```python
from build123d import *

# Parameters (mm, degrees)
BOSS_EXTRUDE1_DEPTH = 4


with BuildPart() as part:
    # Sketch2 → Boss-Extrude1 (new body)
    with BuildSketch(Plane.XY):
        with BuildLine():
            Line((-138.118918248, -4), (-138.118918248, -8))
            Line((-138.118918248, -8), (-118.118918248, -8))
            Line((-118.118918248, -8), (-118.118918248, -4))
            Line((-118.118918248, -4), (-78.118918248, -4))
            Line((-78.118918248, -4), (-78.118918248, -8))
            Line((-78.118918248, -8), (-18.118918248, -8))
            Line((-18.118918248, -8), (-18.118918248, -4))
            Line((-18.118918248, -4), (21.881081752, -4))
            Line((21.881081752, -4), (21.881081752, -8))
            Line((21.881081752, -8), (81.881081752, -8))
            Line((81.881081752, -8), (81.881081752, -4))
            Line((81.881081752, -4), (121.881081752, -4))
            Line((121.881081752, -4), (121.881081752, -8))
            Line((121.881081752, -8), (141.881081752, -8))
            Line((141.881081752, -8), (141.881081752, -4))
            Line((141.881081752, -4), (126.420932439, 77))
            Line((126.420932439, 77), (121.881081752, 77))
            Line((121.881081752, 77), (121.881081752, 47))
            Line((121.881081752, 47), (117.881081752, 47))
            Line((117.881081752, 47), (117.881081752, 77))
            Line((117.881081752, 77), (113.803791589, 77))
            Line((113.803791589, 77), (105.805256721, 36.507417232))
            ThreePointArc((105.805256721, 36.507417232), (101.881081752, 33.282562905), (97.956906783, 36.507417232))
            Line((97.956906783, 36.507417232), (89.958371916, 77))
            Line((89.958371916, 77), (85.881081752, 77))
            Line((85.881081752, 77), (85.881081752, 47))
            Line((85.881081752, 47), (81.881081752, 47))
            Line((81.881081752, 47), (81.881081752, 77))
            Line((81.881081752, 77), (21.881081752, 77))
            Line((21.881081752, 77), (21.881081752, 47))
            Line((21.881081752, 47), (17.881081752, 47))
            Line((17.881081752, 47), (17.881081752, 77))
            Line((17.881081752, 77), (-14.118918248, 77))
            Line((-14.118918248, 77), (-14.118918248, 47))
            Line((-14.118918248, 47), (-18.118918248, 47))
            Line((-18.118918248, 47), (-18.118918248, 77))
            Line((-18.118918248, 77), (-78.118918248, 77))
            Line((-78.118918248, 77), (-78.118918248, 47))
            Line((-78.118918248, 47), (-82.118918248, 47))
            Line((-82.118918248, 47), (-82.118918248, 77))
            Line((-82.118918248, 77), (-86.196208411, 77))
            Line((-86.196208411, 77), (-94.194743279, 36.507417232))
            ThreePointArc((-94.194743279, 36.507417232), (-98.118918248, 33.282562905), (-102.043093217, 36.507417232))
            Line((-102.043093217, 36.507417232), (-110.041628084, 77))
            Line((-110.041628084, 77), (-114.118918248, 77))
            Line((-114.118918248, 77), (-114.118918248, 47))
            Line((-114.118918248, 47), (-118.118918248, 47))
            Line((-118.118918248, 47), (-118.118918248, 77))
            Line((-118.118918248, 77), (-122.658768935, 77))
            Line((-122.658768935, 77), (-138.118918248, -4))
        make_face()
        with BuildLine():
            Line((-102.438497969, 0), (-93.799338527, 0))
            ThreePointArc((-93.799338527, 0), (-90.499180816, 1.739699338), (-90.069664197, 5.445520459))
            Line((-90.069664197, 5.445520459), (-94.389243919, 16.590728056))
            ThreePointArc((-94.389243919, 16.590728056), (-98.118918248, 19.145207598), (-101.848592577, 16.590728056))
            Line((-101.848592577, 16.590728056), (-106.168172299, 5.445520459))
            ThreePointArc((-106.168172299, 5.445520459), (-105.73865568, 1.739699338), (-102.438497969, 0))
        make_face(mode=Mode.SUBTRACT)
        with BuildLine():
            Line((-22.118918248, 4), (-22.118918248, 52.759761907))
            ThreePointArc((-22.118918248, 52.759761907), (-24.865306485, 56.558242859), (-29.333147021, 55.140672109))
            Line((-29.333147021, 55.140672109), (-65.451489175, 6.380910203))
            ThreePointArc((-65.451489175, 6.380910203), (-65.80962942, 2.200505739), (-62.237260401, 0))
            Line((-62.237260401, 0), (-26.118918248, 0))
            ThreePointArc((-26.118918248, 0), (-23.290491123, 1.171572875), (-22.118918248, 4))
        make_face(mode=Mode.SUBTRACT)
        with BuildLine():
            Line((-34.000576095, 73), (-70.118918248, 73))
            ThreePointArc((-70.118918248, 73), (-72.947345373, 71.828427125), (-74.118918248, 69))
            Line((-74.118918248, 69), (-74.118918248, 20.240238093))
            ThreePointArc((-74.118918248, 20.240238093), (-71.372530011, 16.441757141), (-66.904689475, 17.859327891))
            Line((-66.904689475, 17.859327891), (-30.786347321, 66.619089797))
            ThreePointArc((-30.786347321, 66.619089797), (-30.428207076, 70.799494261), (-34.000576095, 73))
        make_face(mode=Mode.SUBTRACT)
        with BuildLine():
            Line((9.881081752, 73), (-2.356754744, 73))
            ThreePointArc((-2.356754744, 73), (-5.664234687, 71.249572499), (-6.076962704, 67.530288213))
            Line((-6.076962704, 67.530288213), (6.160873792, 36.553264583))
            ThreePointArc((6.160873792, 36.553264583), (10.62913528, 34.093546905), (13.881081752, 38.02297637))
            Line((13.881081752, 38.02297637), (13.881081752, 69))
            ThreePointArc((13.881081752, 69), (12.709508877, 71.828427125), (9.881081752, 73))
        make_face(mode=Mode.SUBTRACT)
        with BuildLine():
            Line((-6.118918248, 0), (6.118918248, 0))
            ThreePointArc((6.118918248, 0), (9.426398191, 1.750427501), (9.839126208, 5.469711787))
            Line((9.839126208, 5.469711787), (-2.398710288, 36.446735417))
            ThreePointArc((-2.398710288, 36.446735417), (-6.866971776, 38.906453095), (-10.118918248, 34.97702363))
            Line((-10.118918248, 34.97702363), (-10.118918248, 4))
            ThreePointArc((-10.118918248, 4), (-8.947345373, 1.171572875), (-6.118918248, 0))
        make_face(mode=Mode.SUBTRACT)
        with BuildLine():
            Line((105.610756081, 16.590728056), (109.930335803, 5.445520459))
            ThreePointArc((109.930335803, 5.445520459), (109.500819184, 1.739699338), (106.200661473, 0))
            Line((106.200661473, 0), (97.561502031, 0))
            ThreePointArc((97.561502031, 0), (94.26134432, 1.739699338), (93.831827701, 5.445520459))
            Line((93.831827701, 5.445520459), (98.151407423, 16.590728056))
            ThreePointArc((98.151407423, 16.590728056), (101.881081752, 19.145207598), (105.610756081, 16.590728056))
        make_face(mode=Mode.SUBTRACT)
        with BuildLine():
            Line((70.666852979, 17.859327891), (34.548510825, 66.619089797))
            ThreePointArc((34.548510825, 66.619089797), (34.19037058, 70.799494261), (37.762739599, 73))
            Line((37.762739599, 73), (73.881081752, 73))
            ThreePointArc((73.881081752, 73), (76.709508877, 71.828427125), (77.881081752, 69))
            Line((77.881081752, 69), (77.881081752, 20.240238093))
            ThreePointArc((77.881081752, 20.240238093), (75.134693515, 16.441757141), (70.666852979, 17.859327891))
        make_face(mode=Mode.SUBTRACT)
        with BuildLine():
            Line((65.999423905, 0), (29.881081752, 0))
            ThreePointArc((29.881081752, 0), (27.052654627, 1.171572875), (25.881081752, 4))
            Line((25.881081752, 4), (25.881081752, 52.759761907))
            ThreePointArc((25.881081752, 52.759761907), (28.627469989, 56.558242859), (33.095310525, 55.140672109))
            Line((33.095310525, 55.140672109), (69.213652679, 6.380910203))
            ThreePointArc((69.213652679, 6.380910203), (69.571792924, 2.200505739), (65.999423905, 0))
        make_face(mode=Mode.SUBTRACT)
    extrude(amount=BOSS_EXTRUDE1_DEPTH)


solid = part.part
```
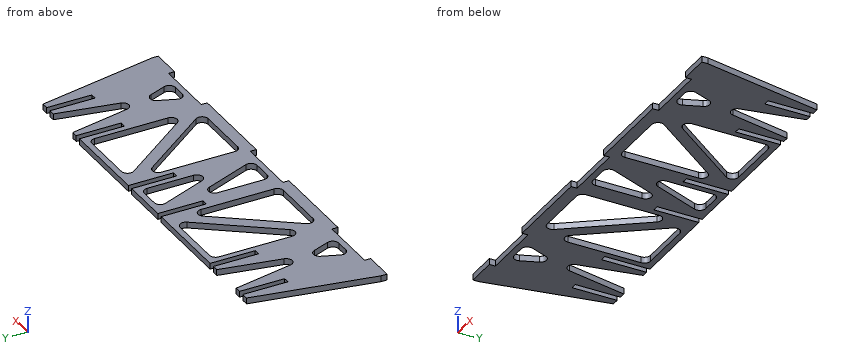
The listing builds one solid part. Answer for the finished solid, in the listing's coordinates (mm). Coordinates: 2 decimals unless noted, no trailing zeros. Write each loop counter-clockwise with the first axis right and the second up, starting at its lowest first coordinate (ties: lowest second). Pieces come first, ordered by that corner, then holes.
Q1. Section C-C, the plane z = 0.9 is taken. Give the number of separate pieces and of enclosed holes in the cut face, then the cut area to 3 significant figures.
Returned:
separate pieces: 1
enclosed holes: 8
area: 12,400 mm2
Q2. Find the intervals of material crossed by line 1 along Y through (x, z) = (44.5, 2.4); line 2 along X through (y, z) = (14, 1.85); line 3 along X through (y, z) = (32, 0.3), in increasing order.
Returned:
line 1: y = -8 to 0, 39.74 to 53.18, 73 to 77
line 2: x = -134.68 to -102.85, -93.39 to -59.81, -22.12 to -10.12, 6.47 to 25.88, 63.57 to 97.15, 106.61 to 138.45
line 3: x = -131.25 to -74.12, -56.43 to -46.47, -22.12 to -10.12, -0.64 to 25.88, 50.24 to 60.19, 77.88 to 135.01
Q3. Section B-B, the plane y = 23.5 is taken. Write down the section's boundary in (x, z).
Returned:
outline: (-132.87, 0) - (-74.12, 0) - (-74.12, 4) - (-132.87, 4) - close; (-62.73, 0) - (-52.77, 0) - (-52.77, 4) - (-62.73, 4) - close; (-22.12, 0) - (-10.12, 0) - (-10.12, 4) - (-22.12, 4) - close; (2.72, 0) - (25.88, 0) - (25.88, 4) - (2.72, 4) - close; (56.53, 0) - (66.49, 0) - (66.49, 4) - (56.53, 4) - close; (77.88, 0) - (136.63, 0) - (136.63, 4) - (77.88, 4) - close
Q4. Section A-A, the plane x = -51.5 is taken. Write down the section's boundary in (y, z).
Returned:
outline: (-8, 0) - (0, 0) - (0, 4) - (-8, 4) - close; (25.22, 0) - (38.66, 0) - (38.66, 4) - (25.22, 4) - close; (73, 0) - (77, 0) - (77, 4) - (73, 4) - close
Q5. Given P1, Ø2, axis at y = 64, z = 2, coming from the +X side; P2, Ø1.2, axis at y = 40.5, z = 1.5, coming from the -X side, each flat-ended and moving along its own axis, determine where each tip first touches the part or whether it passes through.
Returned:
P1: stops at x = 129.09
P2: stops at x = -129.74
